Part model, mm, in its own coordinate system. Give positions to 0.01 mm unless a question says otherwise; leave off trailing zeros. Order: outer loops, then holes, each group sorted by start corner. A loop starts at its lowest first (then second) coordinate and runs counter-clockwise, first axis right, second up. Notation, with made-up numbers: (21.25, -0.5) -> (53.25, -0.5) arc R32 cw to (53.25, 32.5) -> close; hole circle Ø10 at (7, -34). An arc over 180 degrees is marked (long way). Write item = value, one per line. Start each with the question number.
Item 1: Band-saw the part on D-D on x = 25. Write the cut outline in (y, z), plus the area to 3 significant figures.
Item 2: Drill centre lines: line 1 along Y through (x, z) = (-12.7, 4.2); line 2 along Y through (x, z) = (-12.7, 1.05); line 3 along Z through (x, y) = (11.5, -10). Where is each one in solid material? Low to high.
Item 3: Band-saw the part on A-A on x = -12.7. Write the cut outline in (y, z).
Item 4: Band-saw the part on B-B on z = 4.9. Count the separate pieces of the cut face and the enclosed holes in it, plus the area to 3 significant figures.
Item 5: Flat gauge pins, fed straight in: P1, Ø6.5, axis at x = -13, y = 12.5, coming from the +Z side; P2, Ø3, axis at x = 12.7, y = -12.7, coming from the -Z side. Where does each tip first touch, or does it go through?
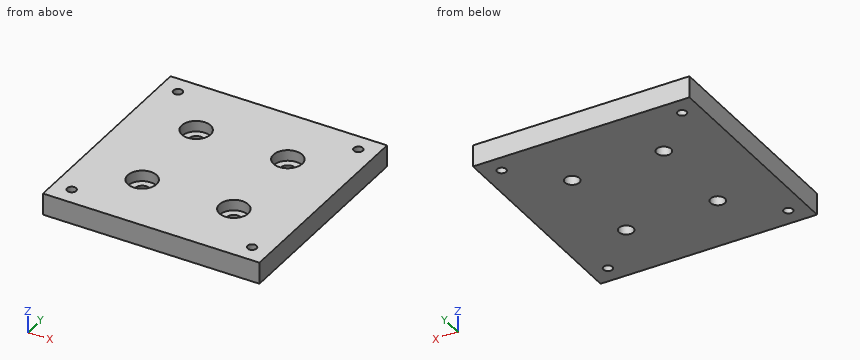
```python
from build123d import *

# Parameters (mm, degrees)
SKETCH_1_W                = 60
SKETCH_1_H                = 60
EXTRUDE_1_DEPTH           = 6
HOLE_WIZARD_M3_1_D        = 2.5
HOLE_WIZARD_1_D           = 4
HOLE_WIZARD_1_CBORE_D     = 8
HOLE_WIZARD_1_CBORE_DEPTH = 3


with BuildPart() as part:
    # 草图1 → 凸台-拉伸1 (new body)
    with BuildSketch(Plane.XY):
        Rectangle(SKETCH_1_W, SKETCH_1_H)
    extrude(amount=EXTRUDE_1_DEPTH)

    # M3 螺纹孔1 (through all)
    with Locations(Plane(origin=(-25, 25, 6), x_dir=(1, 0, 0), z_dir=(0, 0, 1))):
        with Locations((0, 0), (50, 0), (50, -50), (0, -50)):
            Hole(HOLE_WIZARD_M3_1_D / 2)

    # 孔1 (through all)
    with Locations(Plane(origin=(-12.7, 12.7, 6), x_dir=(1, 0, 0), z_dir=(0, 0, 1))):
        with Locations((0, 0), (25.4, 0), (25.4, -25.4), (0, -25.4)):
            CounterBoreHole(HOLE_WIZARD_1_D / 2, HOLE_WIZARD_1_CBORE_D / 2, HOLE_WIZARD_1_CBORE_DEPTH)


solid = part.part
```
Values found:
q1.outline = (-30, 0) -> (-26.25, 0) -> (-26.25, 6) -> (-30, 6) -> close; (-23.75, 0) -> (23.75, 0) -> (23.75, 6) -> (-23.75, 6) -> close; (26.25, 0) -> (30, 0) -> (30, 6) -> (26.25, 6) -> close
q1.area = 330 mm^2
q2.line_1 = -30 to -16.7, -8.7 to 8.7, 16.7 to 30
q2.line_2 = -30 to -14.7, -10.7 to 10.7, 14.7 to 30
q2.line_3 = 0 to 3
q3.outline = (-30, 0) -> (-14.7, 0) -> (-14.7, 3) -> (-16.7, 3) -> (-16.7, 6) -> (-30, 6) -> close; (-10.7, 0) -> (10.7, 0) -> (10.7, 3) -> (8.7, 3) -> (8.7, 6) -> (-8.7, 6) -> (-8.7, 3) -> (-10.7, 3) -> close; (14.7, 0) -> (30, 0) -> (30, 6) -> (16.7, 6) -> (16.7, 3) -> (14.7, 3) -> close
q4.separate_pieces = 1
q4.enclosed_holes = 8
q4.area = 3,380 mm^2
q5.P1 = 3
q5.P2 = through
